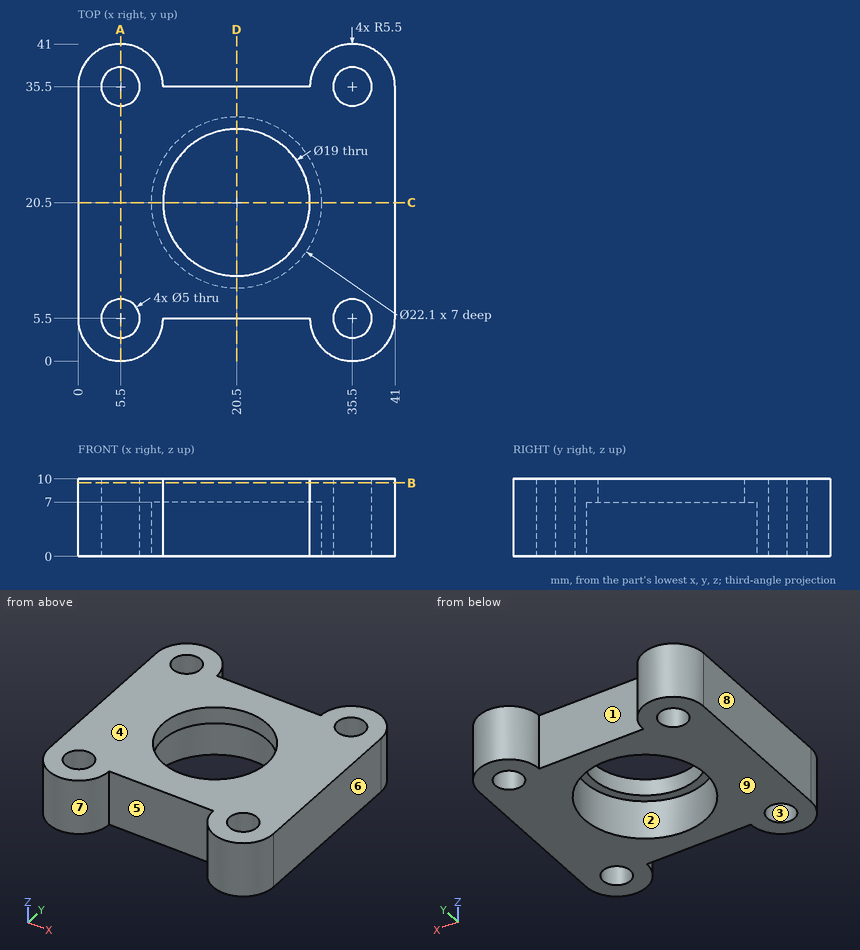
Input: dimensioned drawing with shaded views. Units: mm. Origin: part minimum x, y, z. A direction names the side the tool comes from. Coordinates: 2 decimals unless noted, no trailing zeros. Loops run counter-clockwise (first coordinate to the right, second up) from the corner with the lowest first, then second, coordinate; pieces in that order, holes last.
Q1. Section C-C, the plane y = 20.5. Return the cut outline in (x, z), and give its area (3 significant figures).
Results are:
outline: (0, 0) - (9.45, 0) - (9.45, 7) - (11, 7) - (11, 10) - (0, 10) - close; (30, 7) - (31.55, 7) - (31.55, 0) - (41, 0) - (41, 10) - (30, 10) - close
area: 198 mm2
Q2. Section D-D, the plane x = 20.5. Return the cut outline in (y, z).
Results are:
outline: (5.5, 0) - (9.45, 0) - (9.45, 7) - (11, 7) - (11, 10) - (5.5, 10) - close; (30, 7) - (31.55, 7) - (31.55, 0) - (35.5, 0) - (35.5, 10) - (30, 10) - close
Q3. Mould query, pull axis X, two halves, no side actions, for the marked faces 6, 7, 8 and 9. Classes: +X half, -X half, draft (parallel to the pull), parting line (faces both ways), or undercut.
Results are:
face 6: +X half
face 7: undercut
face 8: -X half
face 9: draft
Q4. Contact query for flat-ended pins moving along their axis: pin 1 (5 mm diameter, centred on x = 19.5, z = 4.5, fed in from +Y); pin 2 (1 mm diameter, centred on x = 10.5, z = 2, fed in from -Y); pin 3 (2 mm diameter, centred on x = 24, z = 4.5, fed in from -Y); pin 4 (17.5 mm diameter, centred on x = 20.5, y = 20.5, fed in from -Z). Output: stop coordinate, or through.
Results are:
pin 1: stops at y = 35.5
pin 2: stops at y = 2.34
pin 3: stops at y = 5.5
pin 4: passes through
Q5. Set-up query: the marked faces 1, 2, 3, 4 and 5. Return all of +Z, -Z, +X, -X, +Y, -Y with unobstructed straight access to the full face (end or side cutting, diameter ignored); none if empty.
Results are:
face 1: +Z, -Z, +Y
face 2: -Z
face 3: +Z, -Z
face 4: +Z, +X, -X, +Y, -Y
face 5: +Z, -Z, -Y
Q6. Line query: line 1 along Y through (x, z) = (35.5, 4.5); line 2 along Y through (x, z) = (20.5, 2); line 3 along X through (y, z) = (20.5, 2.75). Output: solid intervals per line, ascending.
Results are:
line 1: y = 0 to 3, 8 to 33, 38 to 41
line 2: y = 5.5 to 9.45, 31.55 to 35.5
line 3: x = 0 to 9.45, 31.55 to 41
Q7. Section A-A, the plane x = 5.5. Return the cut outline in (y, z).
Results are:
outline: (0, 0) - (3, 0) - (3, 10) - (0, 10) - close; (8, 0) - (33, 0) - (33, 10) - (8, 10) - close; (38, 0) - (41, 0) - (41, 10) - (38, 10) - close
Q8. Section B-B, the plane z = 9.5. Return the cut outline in (x, y), and give its area (3 significant figures).
Results are:
outline: (0, 5.5) arc R5.5 ccw to (11, 5.5) - (30, 5.5) arc R5.5 ccw to (41, 5.5) - (41, 35.5) arc R5.5 ccw to (30, 35.5) - (11, 35.5) arc R5.5 ccw to (0, 35.5) - close; hole circle Ø5 at (5.5, 5.5); hole circle Ø5 at (5.5, 35.5); hole circle Ø19 at (20.5, 20.5); hole circle Ø5 at (35.5, 5.5); hole circle Ø5 at (35.5, 35.5)
area: 1,060 mm2
